from build123d import *

# Parameters (mm, degrees)
SKETCH1_W           = 100
SKETCH1_H           = 120
BOSS_EXTRUDE1_DEPTH = 20
SKETCH2_W           = 90
SKETCH2_H           = 110
CUT_EXTRUDE1_DEPTH  = 16
SKETCH4_W           = 5
SKETCH4_H           = 5
SKETCH4_W_2         = 70
CUT_EXTRUDE2_DEPTH  = 121


with BuildPart() as part:
    # Sketch1 → Boss-Extrude1 (new body)
    with BuildSketch(Plane(origin=(0, 0, 0), x_dir=(1, 0, 0), z_dir=(0, 1, 0))):
        Rectangle(SKETCH1_W, SKETCH1_H)
    extrude(amount=BOSS_EXTRUDE1_DEPTH)

    # Sketch2 → Cut-Extrude1 (cut)
    with BuildSketch(Plane(origin=(0, 20, 0), x_dir=(1, 0, 0), z_dir=(0, 1, 0))):
        Rectangle(SKETCH2_W, SKETCH2_H)
    extrude(amount=-CUT_EXTRUDE1_DEPTH, mode=Mode.SUBTRACT)

    # Sketch4 → Cut-Extrude2 (cut, through all)
    with BuildSketch(Plane.XY.offset(60)):
        with Locations((-47.5, 17.5)):
            Rectangle(SKETCH4_W, SKETCH4_H)
        with Locations((47.5, 17.5)):
            Rectangle(SKETCH4_W, SKETCH4_H)
        with Locations((0, 17.5)):
            Rectangle(SKETCH4_W_2, SKETCH4_H)
    extrude(amount=-CUT_EXTRUDE2_DEPTH, mode=Mode.SUBTRACT)


solid = part.part
Can you work these out from the model? Positions are in its coordinate system, mm. A direction names the side the tool comes from. Give positions to 0.01 mm unless a question says otherwise; leave off trailing zeros. Order: outer loops, then holes, each group sorted by start corner. A loop starts at its lowest first (then second) coordinate and runs counter-clockwise, first axis right, second up. Notation, with made-up numbers: M 60,-24.75 L 64,-24.75 A19 ccw 64,-20.75 Z; hole C 55.5,83 d1. An arc over 180 degrees is marked long. One line per question, with ' | ' between items.
Item 1: We'd pull the mould along Z, two halves only. Please class faces 1 (the face through (-45, 10, 1)), 2 (the face through (45, 17, 58)), 3 (the face through (45, 10, 1)), 4 (the face through (-1, 8, -60)): released by +Z, released by -Z, zero draft, split by the parting line, or undercut.
Answer block:
face 1: undercut | face 2: zero draft | face 3: undercut | face 4: released by -Z
Item 2: I'm going to push flat-ended pins straight in: pin 1 Ø2.5 at (y, z) = (16.5, -57) entering from +X; pin 2 Ø2.5 at (y, z) = (17, -58.5) entering from -X; pin 3 Ø8 at (x, z) = (10.5, -42.5) entering from +Y; pin 4 Ø5.5 at (y, z) = (16.5, 56.5) entering from -X. Where does each tip first touch, or does it pass through?
Answer block:
pin 1: stops at x = 45 | pin 2: stops at x = -45 | pin 3: stops at y = 4 | pin 4: stops at x = -50
Item 3: Suppose I cut it at C-C, the plane x = -40. Write out the boundary of the cut face in (y, z), then the cut area to 3 significant figures.
Answer block:
outline: M 0,-60 L 20,-60 L 20,-55 L 4,-55 L 4,55 L 20,55 L 20,60 L 0,60 Z | area: 640 mm2
Item 4: For faces 5 (the face through (-45, 17, -57)), 6 (the face through (0, 15, 58)), 7 (the face through (-1, 10, -55)), which set-ups out of +Z, -Z, +X, -X, +Y, -Y let a thin tool reach every point of the face, with its end or its side?
Answer block:
face 5: +Z, -Z, -X, +Y | face 6: +Z, -Z, +Y | face 7: +Y
Item 5: Suppose I cut it at B-B, the plane z = -15.5. Write out the boundary of the cut face in (x, y).
Answer block:
outline: M -50,0 L 50,0 L 50,15 L 45,15 L 45,4 L -45,4 L -45,15 L -50,15 Z
Item 6: Suppose I cut it at A-A, the plane y = 17.75. Write out the boundary of the cut face in (x, z), then the cut area to 3 significant figures.
Answer block:
outline: M -45,-60 L -35,-60 L -35,-55 L -45,-55 Z; M -45,55 L -35,55 L -35,60 L -45,60 Z; M 35,-60 L 45,-60 L 45,-55 L 35,-55 Z; M 35,55 L 45,55 L 45,60 L 35,60 Z | area: 200 mm2
Item 7: Please list where these lines run through material, in increasing order: L1, parallel to X at y = 14, z = -12; L2, parallel to Z at x = -39, y = 13.5; L3, parallel to Y at x = 9.5, z = -34.
Answer block:
L1: x = -50 to -45, 45 to 50 | L2: z = -60 to -55, 55 to 60 | L3: y = 0 to 4
